Geometry check sheet. Reference: the model listing, model coordinates, mm. A direction names the side the tool comes from. Coordinates: 2 decimals unless noted, no trailing zeros. Order: outer loops, then holes, each group sorted by start corner. A loop starts at its lowest first (then second) coordinate and runs counter-clockwise, first axis right, second up. Notation, with made-up numbers: M 44.5,14.25 L 96.5,14.25 A22 cw 96.5,36.25 Z; hole C -23,14 d10. An arc over 180 degrees is marked long. One line per item, written item: value. Start each with the question number.
1) Thickness scan on L1, parallel to Y at x = 0, z = -81.5; L2, parallel to Y at x = 0, z = -85.3; L3, parallel to Z at x = 6, y = 12. Record the ranges inside material, lowest first. Write a range as from..to.
2) Access from +Z, -Z, +X, -X, +Y, -Y to the whole of each face (thin tool, end or side, straight path). Record for faces 1 (the cylindrical face through (-1.98, -15.11, -85.07)), 2 (the cylindrical face through (3.78, -2.9, -85.63)).
3) Draft check along X on faces 3 (the flat face through (-2, -2, -84.887)), 4 (the flat face through (-3.5, -12.5, -83.82)), 5 (the cylindrical face through (5.86, 11.267, -77.382)). Enter one of: pulls with the +X half, pulls with the -X half, needs draft (parallel to the pull), parting line crosses it, or undercut.
4) Go/stop test with flat-tipped pins: P1, Ø4, axis at x = 11.5, z = -73.5, coming from the +Y side; P2, Ø1.5, axis at y = -10.5, z = -80.5, coming from the -X side; P3, Ø1, axis at x = -1, z = -81, coming from the +Y side. Record where each tip stops, or that it passes through.
5) Sectioned sample at A-A, the plane y = 0. Enter the section's corners in (x, z), then the cut area to 3 significant figures.
6) Sectioned sample at D-D, the plane y = -5.5. Enter the section's corners in (x, z), then the cut area to 3 significant figures.
7) Sectioned sample at C-C, the plane z = -73.5. Enter the section's corners in (x, y).
```python
from build123d import *

# Parameters (mm, degrees)
SKETCH2_R          = 2.5796875
CUT_EXTRUDE1_DEPTH = 27.396454307
SKETCH3_R          = 4.7625
CUT_EXTRUDE2_DEPTH = 1.4732


with BuildPart() as part:
    # Sketch1 → Revolve1 (revolve)
    with BuildSketch(Plane(origin=(0, 0, 0), x_dir=(1, 0, 0), z_dir=(0, 1, 0)), mode=Mode.PRIVATE) as revolve1_sk:
        Polygon((0, 71.120493703), (0, 86.360493703), (-15.24, 86.360493703), (-15.24, 83.820493703), (-12.7, 83.820493703), (-12.7, 71.120493703), align=None)
    revolve(revolve1_sk.sketch.rotate(Axis((0, 0, 0), (0, 0, -1)), 180), axis=Axis((0, 0, 0), (0, 0, -1)))

    # Sketch2 → Cut-Extrude1 (cut, through all)
    with BuildSketch(Plane(origin=(0, 0, -86.360493703), x_dir=(-1, 0, 0), z_dir=(0, 0, -1))):
        Circle(SKETCH2_R)
    extrude(amount=-CUT_EXTRUDE1_DEPTH, mode=Mode.SUBTRACT)

    # Sketch3 → Cut-Extrude2 (cut)
    with BuildSketch(Plane(origin=(0, 0, -86.360493703), x_dir=(-1, 0, 0), z_dir=(0, 0, -1))):
        Circle(SKETCH3_R)
    extrude(amount=-CUT_EXTRUDE2_DEPTH, mode=Mode.SUBTRACT)


solid = part.part
```
Final values:
1. L1: y = -12.7..-2.58, 2.58..12.7
1. L2: y = -15.24..-4.76, 4.76..15.24
1. L3: z = -86.36..-83.82
2. face 1: +Z, -Z
2. face 2: -Z
3. face 3: undercut
3. face 4: needs draft
3. face 5: parting line crosses it
4. P1: stops at y = 8.43
4. P2: stops at x = -8.14
4. P3: stops at y = 12.69
5. outline: M -15.24,-86.36 L -4.76,-86.36 L -4.76,-84.89 L -2.58,-84.89 L -2.58,-71.12 L -12.7,-71.12 L -12.7,-83.82 L -15.24,-83.82 Z; M 2.58,-84.89 L 4.76,-84.89 L 4.76,-86.36 L 15.24,-86.36 L 15.24,-83.82 L 12.7,-83.82 L 12.7,-71.12 L 2.58,-71.12 Z
5. area: 315 mm^2
6. outline: M -14.21,-86.36 L 14.21,-86.36 L 14.21,-83.82 L 11.45,-83.82 L 11.45,-71.12 L -11.45,-71.12 L -11.45,-83.82 L -14.21,-83.82 Z
6. area: 363 mm^2
7. outline: C 0,0 d25.4; hole C 0,0 d5.16
